Model file for the job. Use its own axes, mm. Face numbers are marked on the shaded views. A direction names the side the tool comes from. Give positions to 0.01 mm unless a question says otherwise; leave off trailing zeros. Order: outer loops, then holes, each group sorted by start corner. A loop starts at its lowest first (then second) coordinate and runs counter-clockwise, first axis right, second up. Notation, with made-up numbers: (36, -27.75) -> (45, -27.75) arc R17 ccw to (45, -11.75) -> close; hole circle Ø5 at (88, 31.5). An arc over 180 degrees is marked (long way). Use CSV: the item, a comma, the result in double quotes. Start each with the question number.
1. Cut at A-A on y = -27.5. List the corners of the cut face in (x, z).
2. Drop flat-ended pins along their axis: pin 1 (5 mm diameter, centred on x = -7.46, z = -10.5, fed in from +Y); pin 2 (5 mm diameter, centred on x = -1, z = -12.5, fed in from +Y); pin 3 (2.5 mm diameter, centred on x = 7.54, z = -10.44, fed in from -Y). Give the stop position or say it passes through.
3. Pull direction Z, two halves, no side cores. Call the marked faces 1, 2 and 3: released by +Z, released by -Z, zero draft, split by the parting line, or undercut.
4. Cut at C-C on z = -4.5. List the corners of the cut face in (x, y), then the cut area to 3 significant figures.
5. Wall check: line 1 (X direction, y = -44.35, z = -10.5); line 2 (X direction, y = -23.25, z = -18.5); line 3 (X direction, y = -24, z = -5.5). Give the ranges that are in metal, low to high. Write a range as from..to.
6. 3-axis set-ups, long thin cutter, end or side, ignore diameter. For the marked faces 4 and 5: which of +Z, -Z, +X, -X, +Y, -Y reach the whole face in a straight line?
7. Cut at D-D on x = -7. List the corners of the cut face in (y, z), then the cut area to 3 significant figures.
8. Cut at B-B on x = 11.25. List the corners of the cut face in (y, z).
```python
from build123d import *

# Parameters (mm, degrees)
BOSS_EXTRUDE4_DEPTH = 21
SKETCH7_R           = 1.6
CUT_EXTRUDE1_DEPTH  = 3
SKETCH5_R           = 1.85
BOSS_EXTRUDE5_DEPTH = 3
BOSS_EXTRUDE6_START = 3
SKETCH8_R           = 1.85
BOSS_EXTRUDE6_DEPTH = 3


with BuildPart() as part:
    # Sketch1 → Boss-Extrude4 (new body)
    with BuildSketch(Plane.XY):
        Polygon((12.320696932, -20.271970514), (14.320696932, -20.271970514), (14.320696932, -45.271970514), (-14.239524115, -45.271970514), (-14.239524115, -20.271970514), (-12.239524115, -20.271970514), (-12.239524115, -43.271970514), (12.320696932, -43.271970514), align=None)
    extrude(amount=-BOSS_EXTRUDE4_DEPTH)

    # Sketch7 → Cut-Extrude1 (cut)
    with BuildSketch(Plane.XZ.offset(45.271970514)):
        with Locations(Location((-7.459347, -10.5, 0), (0, 0, 270))):
            Circle(SKETCH7_R)
        with Locations(Location((7.540540263, -10.441844196, 0), (0, 0, 90))):
            Circle(SKETCH7_R)
    extrude(amount=-CUT_EXTRUDE1_DEPTH, mode=Mode.SUBTRACT)

    # Sketch5 → Boss-Extrude5 (add)
    with BuildSketch(Plane(origin=(-12.239524115, 0, 0), x_dir=(0, 0, -1), z_dir=(1, 0, 0))):
        with Locations((16.5, -24)):
            Circle(SKETCH5_R)
        with Locations((10.5, -24)):
            Circle(SKETCH5_R)
        with Locations((4.5, -24)):
            Circle(SKETCH5_R)
    extrude(amount=BOSS_EXTRUDE5_DEPTH)

    # Sketch8 → Boss-Extrude6 (add)
    with BuildSketch(Plane.ZY.offset(-12.320696932).offset(BOSS_EXTRUDE6_START)):
        with Locations(Location((-16.5, -24, 0), (0, 0, 180))):
            Circle(SKETCH8_R)
        with Locations(Location((-10.5, -24, 0), (0, 0, 180))):
            Circle(SKETCH8_R)
        with Locations(Location((-4.5, -24, 0), (0, 0, 180))):
            Circle(SKETCH8_R)
    extrude(amount=-BOSS_EXTRUDE6_DEPTH)


solid = part.part
```
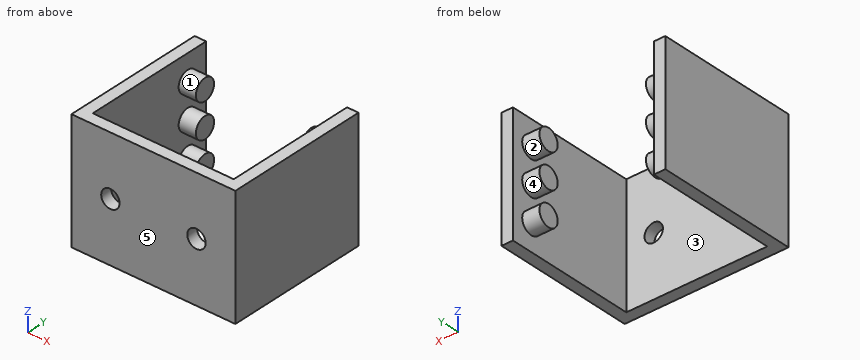
Verdict:
1,outline,"(-14.24, -21) -> (-12.24, -21) -> (-12.24, 0) -> (-14.24, 0) -> close; (12.32, -21) -> (14.32, -21) -> (14.32, 0) -> (12.32, 0) -> close"
2,pin 1,"y = -22.15"
2,pin 2,"y = -43.27"
2,pin 3,"through"
3,face 1,"undercut"
3,face 2,"undercut"
3,face 3,"zero draft"
4,outline,"(-14.24, -45.27) -> (14.32, -45.27) -> (14.32, -20.27) -> (12.32, -20.27) -> (12.32, -22.15) -> (9.32, -22.15) -> (9.32, -25.85) -> (12.32, -25.85) -> (12.32, -43.27) -> (-12.24, -43.27) -> (-12.24, -25.85) -> (-9.24, -25.85) -> (-9.24, -22.15) -> (-12.24, -22.15) -> (-12.24, -20.27) -> (-14.24, -20.27) -> close"
4,area,"171 mm^2"
5,line 1,"-14.24..-9.06, -5.86..5.94, 9.14..14.32"
5,line 2,"-14.24..-12.24, 12.32..14.32"
5,line 3,"-14.24..-9.24, 9.32..14.32"
6,face 4,"none"
6,face 5,"+Z, -Z, +X, -X, -Y"
7,outline,"(-45.27, -21) -> (-43.27, -21) -> (-43.27, -12.03) -> (-45.27, -12.03) -> close; (-45.27, -8.97) -> (-43.27, -8.97) -> (-43.27, 0) -> (-45.27, 0) -> close"
7,area,"35.9 mm^2"
8,outline,"(-45.27, -21) -> (-43.27, -21) -> (-43.27, 0) -> (-45.27, 0) -> close; circle Ø3.7 at (-24, -16.5); circle Ø3.7 at (-24, -10.5); circle Ø3.7 at (-24, -4.5)"
